The listing builds one solid part. Answer for the finished solid, in the listing's coordinates (mm). Coordinates: 2 decimals unless noted, no trailing zeros. Loops run counter-clockwise (first coordinate to the right, second up) from the corner with the lowest first, then second, coordinate; pieces in that order, holes last. Notation, with made-up numbers: M -27,76 L -14,76 A28 cw -14,99 Z; hole C 20.5,-5.5 d5. An arc over 180 degrees is marked long. Return JSON: item names as keys, results as strings. Group by question number.
1. Section D-D (y = -2.75) is taken. Write down the section's boundary in (x, z), then the cut area to 3 significant figures.
2. Section B-B (z = 5) is taken. Write down the section's boundary in (x, y).
3. Straight lines are drawn through the part: L1, parallel to X at y = -10.25, z = 37.5; L2, parallel to X at y = -3.75, z = 38.5; L3, parallel to Z at x = 20.5, y = -11.25. For each, find the intervals that lie inside material, in ascending order. Write a range as from..to.
4. Given P1, Ø10.5, axis at x = -8.23, z = 36.06, coming from the -Y side; P2, Ø4, axis at x = 38, y = -12, coming from the -Z side; P3, Ø6, axis at x = -27.5, z = -9, coming from the +Y side, each flat-ended and moving along its own axis, determine where each tip first touches the part or whether it passes through.
5. Section A-A (x = -9.5) is taken. Write down the section's boundary in (y, z).
6. Section C-C (z = 31.5) is taken. Write down the section's boundary in (x, y), then the cut area to 3 significant figures.
```python
from build123d import *

# Parameters (mm, degrees)
F1_DEPTH = 15
F2_R     = 8.89
F3_DEPTH = 508


with BuildPart() as f1:
    # F0 (on Front) → F1 (new body)
    with BuildSketch(Plane.XZ):
        Polygon((57.845067, 46.221994), (-43.789256, 46.221994), (-43.789256, -55.412333), (-18.380675, -55.412333), (57.845067, 20.813413), align=None)
    extrude(amount=F1_DEPTH)

    # F2 (on face) → F3 (cut)
    with BuildSketch(Plane.XZ.offset(15)):
        with Locations((-33.629256, 36.061994)):
            Circle(F2_R)
        with Locations((-33.629256, 10.661994)):
            Circle(F2_R)
        with Locations((-33.629256, -14.738006)):
            Circle(F2_R)
        with Locations((-33.629256, -40.138006)):
            Circle(F2_R)
        with Locations((-8.229256, 36.061994)):
            Circle(F2_R)
        with Locations((17.170744, 36.061994)):
            Circle(F2_R)
        with Locations((42.570744, 36.061994)):
            Circle(F2_R)
    extrude(amount=-F3_DEPTH, mode=Mode.SUBTRACT)


solid = f1.part
```
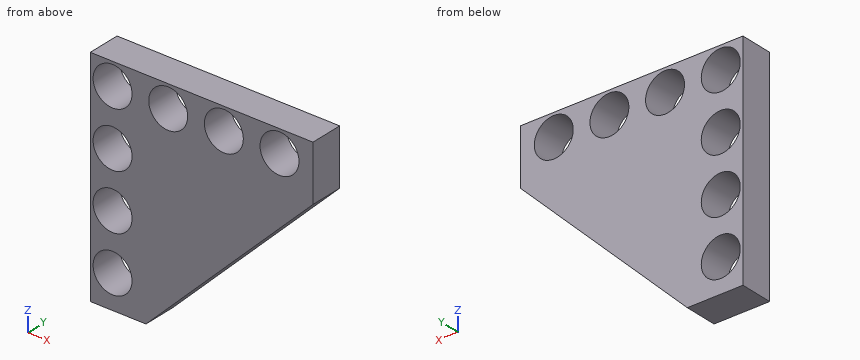
Worked out:
{
 "1": {"outline": "M -43.79,-55.41 L -18.38,-55.41 L 57.85,20.81 L 57.85,46.22 L -43.79,46.22 Z; hole C -33.63,-40.14 d17.78; hole C -33.63,-14.74 d17.78; hole C -33.63,10.66 d17.78; hole C -33.63,36.06 d17.78; hole C -8.23,36.06 d17.78; hole C 17.17,36.06 d17.78; hole C 42.57,36.06 d17.78", "area": "5,690 mm^2"},
 "2": {"outline": "M -43.79,-15 L -40.48,-15 L -40.48,0 L -43.79,0 Z; M -26.78,-15 L 42.03,-15 L 42.03,0 L -26.78,0 Z"},
 "3": {"L1": "-43.79..-42.4, -24.86..-17, 0.54..8.4, 25.94..33.8, 51.34..57.85", "L2": "-43.79..-42.18, -25.08..-16.78, 0.32..8.62, 25.72..34.02, 51.12..57.85", "L3": "-16.53..27.82, 44.31..46.22"},
 "4": {"P1": "through", "P2": "z = -1.03", "P3": "y = 0"},
 "5": {"outline": "M -15,-46.53 L 0,-46.53 L 0,27.26 L -15,27.26 Z; M -15,44.86 L 0,44.86 L 0,46.22 L -15,46.22 Z"},
 "6": {"outline": "M -43.79,-15 L -41.26,-15 L -41.26,0 L -43.79,0 Z; M -26,-15 L -15.86,-15 L -15.86,0 L -26,0 Z; M -0.6,-15 L 9.54,-15 L 9.54,0 L -0.6,0 Z; M 24.8,-15 L 34.94,-15 L 34.94,0 L 24.8,0 Z; M 50.2,-15 L 57.85,-15 L 57.85,0 L 50.2,0 Z", "area": "609 mm^2"}
}
